The figure shows three views and two pictorial views of one solid part (mm, origin at its lowest corner). Answer the questions. A direction names the side the tool comes from. Give positions to 0.01 mm unless a question says otherwise; leave off trailing zeros. Loops run counter-clockwise (first coordinate to the right, second up) from the corner with the lowest first, then second, coordinate; pieces in that order, holes last. Notation, with made-up numbers: (9.25, 31.5) - (21.25, 31.5) arc R20 cw to (21.25, 65.5) - close; hole circle Ø3 at (-3.5, 24). An arc over 180 degrees is marked (long way). One line per question, with ' | ' between items.
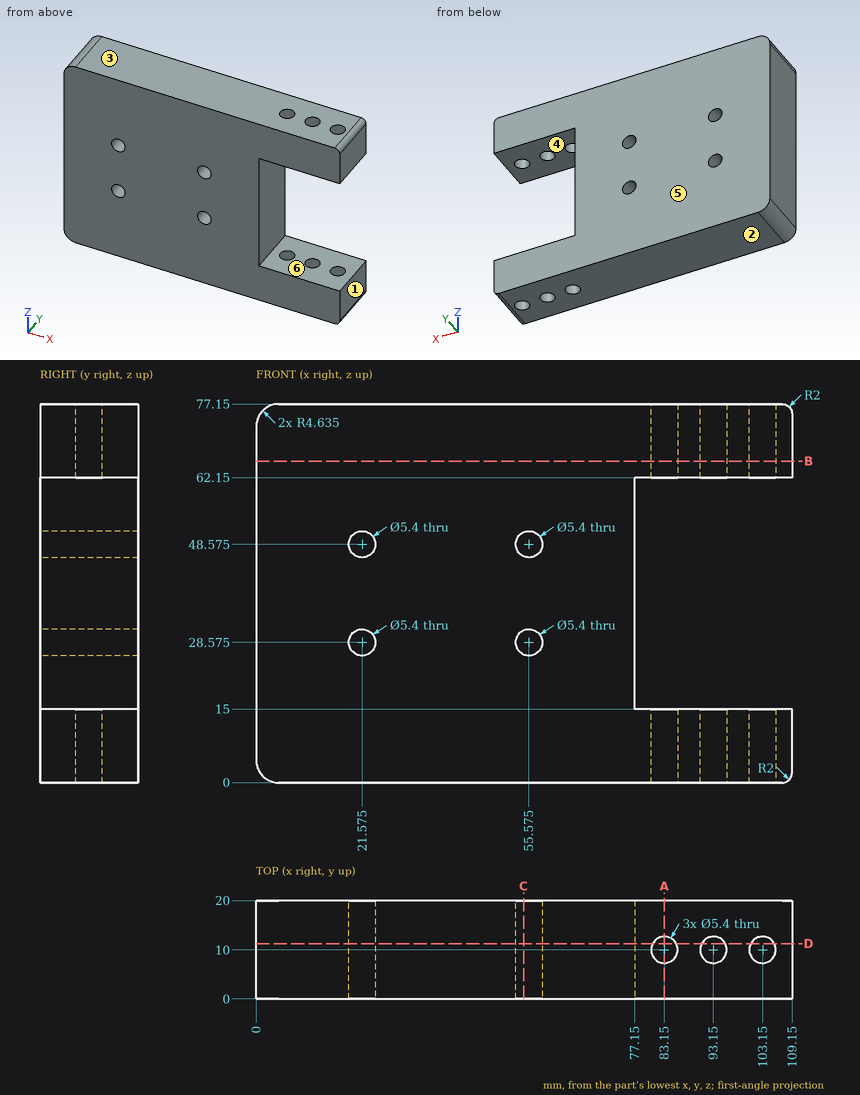
1. Determine the mould class of the marked faces 1, 2, 3 and 4 for opening direction Z: +Z half, -Z half, draft (parallel to the pull), parting line (faces both ways), or undercut.
Evaluation:
face 1: draft | face 2: -Z half | face 3: +Z half | face 4: undercut
2. Find section A-A on x = 83.15. Write down the section's boundary in (y, z), then the cut area to 3 significant figures.
Evaluation:
outline: (0, 0) - (7.3, 0) - (7.3, 15) - (0, 15) - close; (0, 62.15) - (7.3, 62.15) - (7.3, 77.15) - (0, 77.15) - close; (12.7, 0) - (20, 0) - (20, 15) - (12.7, 15) - close; (12.7, 62.15) - (20, 62.15) - (20, 77.15) - (12.7, 77.15) - close | area: 438 mm2
3. Find section B-B on z = 65.5. Write down the section's boundary in (x, y).
Evaluation:
outline: (0, 0) - (109.15, 0) - (109.15, 20) - (0, 20) - close; hole circle Ø5.4 at (83.15, 10); hole circle Ø5.4 at (93.15, 10); hole circle Ø5.4 at (103.15, 10)
4. Find section C-C on x = 54.5. Write down the section's boundary in (y, z).
Evaluation:
outline: (0, 0) - (20, 0) - (20, 26.1) - (0, 26.1) - close; (0, 31.05) - (20, 31.05) - (20, 46.1) - (0, 46.1) - close; (0, 51.05) - (20, 51.05) - (20, 77.15) - (0, 77.15) - close
5. Consider L1, parallel to Y at x = 83.15, z = 8; L2, parallel to Z at x = 78, y = 7.25; L3, parallel to Z at x = 54, y = 10.5. Determine where each line is inside the solid, lowest interval first.
Evaluation:
L1: 0 to 7.3, 12.7 to 20 | L2: 0 to 15, 62.15 to 77.15 | L3: 0 to 26.38, 30.77 to 46.38, 50.77 to 77.15
6. A flat-ended cylindrical pin translates along its axis: pin 1 (6 mm diameter, centred on y = 11, z = 45.5, fed in from +X). Find the tip coordinate at first contact, or state that the pin passes through.
Evaluation:
pin 1: x = 77.15
7. Which of the six approach directions +Z, -Z, +X, -X, +Y, -Y give full straight-line access (tool end or side, diameter ignored) to the marked faces 5 and 6?
Evaluation:
face 5: +Z, -Z, +X, -X, +Y | face 6: +X, +Y, -Y
8. Find section D-D on y = 11.25. State how many separate pieces and enclosed holes the cut face has, then the cut area to 3 significant figures.
Evaluation:
separate pieces: 7 | enclosed holes: 4 | area: 6,380 mm2
